```python
from build123d import *

# Parameters (mm, degrees)
SKETCH1_R           = 13.8327
SKETCH1_R_2         = 13.15
BOSS_EXTRUDE1_DEPTH = 3
BOSS_EXTRUDE2_START = 2
SKETCH2_R           = 13.8327
SKETCH2_R_2         = 9.025
BOSS_EXTRUDE2_DEPTH = 2
BOSS_EXTRUDE3_START = 3
SKETCH3_R           = 13.8327
SKETCH3_R_2         = 13.15
BOSS_EXTRUDE3_DEPTH = 3
FILLET1_R           = 0.5
SKETCH4_R           = 9.525
CUT_EXTRUDE2_DEPTH  = 1.5


with BuildPart() as part:
    # Sketch1 → Boss-Extrude1 (new body)
    with BuildSketch(Plane.XY):
        Circle(SKETCH1_R)
        Circle(SKETCH1_R_2, mode=Mode.SUBTRACT)
    extrude(amount=-BOSS_EXTRUDE1_DEPTH)

    # Sketch2 → Boss-Extrude2 (add)
    with BuildSketch(Plane.XY.offset(BOSS_EXTRUDE2_START)):
        Circle(SKETCH2_R)
        Circle(SKETCH2_R_2, mode=Mode.SUBTRACT)
    extrude(amount=-BOSS_EXTRUDE2_DEPTH)

    # Sketch3 → Boss-Extrude3 (add)
    with BuildSketch(Plane.XY.offset(2).offset(BOSS_EXTRUDE3_START)):
        Circle(SKETCH3_R)
        Circle(SKETCH3_R_2, mode=Mode.SUBTRACT)
    extrude(amount=-BOSS_EXTRUDE3_DEPTH)

    # Fillet1
    fillet1_edges = [part.edges().sort_by_distance(p)[0] for p in [
        (-13.15, 0, 0),
        (-13.15, 0, 2),
    ]]
    fillet(fillet1_edges, radius=FILLET1_R)

    # Sketch4 → Cut-Extrude2 (cut)
    with BuildSketch(Plane(origin=(0, 0, 0), x_dir=(-1, 0, 0), z_dir=(0, 0, -1))):
        Circle(SKETCH4_R)
    extrude(amount=-CUT_EXTRUDE2_DEPTH, mode=Mode.SUBTRACT)


solid = part.part
```
Source: CAD feature listing. Evaluate the final solid. Frame: model axes, mm. A direction names the side the tool comes from. Coordinates: 2 decimals unless noted, no trailing zeros. Loops run counter-clockwise (first coordinate to the right, second up) from the corner with the lowest first, then second, coordinate; pieces in that order, holes last. Notation, with made-up numbers: M -28,-11 L 14,-11 A15 cw 14,12 Z; hole C 40,81 d11. An arc over 180 degrees is marked long. Use CSV: the item, a comma, the result in double quotes.
(1) Draft query along X for faces 1 (the face through (-9, 3, 2)), 2 (the face through (-0.1, -13.3, 5)), 3 (the face through (-2.999, -13.504, 1.056)). Return one class per face: pulls with the +X half, pulls with the -X half, needs draft (parallel to the pull), parting line crosses it, or undercut.
Answers follow:
face 1,"undercut"
face 2,"needs draft"
face 3,"parting line crosses it"
(2) Contact query for flat-ended pins moving along their axis: pin 1 (8 mm diameter, centred on x = -5.5, y = -7, fed in from +Z); pin 2 (4 mm diameter, centred on y = 8, z = 1.5, fed in from +X); pin 3 (9.5 mm diameter, centred on x = -4, y = -2.5, fed in from -Z). Output: stop coordinate, or through.
Answers follow:
pin 1,"z = 2.07"
pin 2,"x = 12.46"
pin 3,"z = 1.5"
(3) Reachability of faces 4 (the face through (-13.137, 0.578, 3.768)), 5 (the face through (7.559, -5.796, 0.74)), 6 (the face through (-0.1, -13.3, -3)) from +Z, -Z, +X, -X, +Y, -Y: full face, straight path, thin tool, end or side. Return the list, or none.
Answers follow:
face 4,"+Z"
face 5,"-Z"
face 6,"-Z, +X, -X, +Y, -Y"
(4) Line query: line 1 (Y direction, x = 0, z = 1.85) (3 decimals); line 2 (Y direction, x = 0, z = -1.6); line 3 (Z direction, x = -11.25, y = -0.75). Output: solid intervals per line, ascending. Write a range as [from, to].
Answers follow:
line 1,"[-13.833, -9.025], [9.025, 13.833]"
line 2,"[-13.83, -13.15], [13.15, 13.83]"
line 3,"[0, 2]"
(5) Cut plane C-C on z = 3.25. Return loops of the section in (x, y), and give its area (3 significant figures).
Answers follow:
outline,"C 0,0 d27.67; hole C 0,0 d26.3"
area,"57.9 mm²"
(6) Cut plane A-A on y = 0. Return loops of the section in (x, z) (3 decimals), and give its area (3 significant figures).
Answers follow:
outline,"M -13.833,-3 L -13.15,-3 L -13.15,-0.5 A0.5 cw -12.65,0 L -9.525,0 L -9.525,1.5 L -9.025,1.5 L -9.025,2 L -12.65,2 A0.5 cw -13.15,2.5 L -13.15,5 L -13.833,5 Z; M 9.025,1.5 L 9.525,1.5 L 9.525,0 L 12.65,0 A0.5 cw 13.15,-0.5 L 13.15,-3 L 13.833,-3 L 13.833,5 L 13.15,5 L 13.15,2.5 A0.5 cw 12.65,2 L 9.025,2 Z"
area,"26.1 mm²"
